Source: CAD feature listing. Evaluate the final solid. Frame: model axes, mm. A direction names the side the tool comes from. Coordinates: 2 decimals unless noted, no trailing zeros. Order: outer loops, then holes, each group sorted by start corner. A loop starts at its lowest first (then second) coordinate and runs counter-clockwise, first axis right, second up.
```python
from build123d import *

# Parameters (mm, degrees)
SKETCH1_W                 = 50.8
SKETCH1_H                 = 50.8
BOSS_EXTRUDE1_DEPTH       = 15.875
SKETCH2_R                 = 3.175
CUT_EXTRUDE1_DEPTH        = 59.973007597
TAP_DRILL_FOR_8_32_TAP1_D = 3.4544
SKETCH5_R                 = 3.81
CUT_EXTRUDE2_DEPTH        = 6.35


with BuildPart() as part:
    # Sketch1 → Boss-Extrude1 (new body)
    with BuildSketch(Plane(origin=(0, 0, 0), x_dir=(1, 0, 0), z_dir=(0, 1, 0))):
        Rectangle(SKETCH1_W, SKETCH1_H)
    extrude(amount=BOSS_EXTRUDE1_DEPTH)

    # Sketch2 → Cut-Extrude1 (cut, through all)
    with BuildSketch(Plane.XY.offset(25.4)):
        with Locations((-19.05, 7.9375)):
            Circle(SKETCH2_R)
        with Locations((0, 7.9375)):
            Circle(SKETCH2_R)
        with Locations((19.05, 7.9375)):
            Circle(SKETCH2_R)
    extrude(amount=-CUT_EXTRUDE1_DEPTH, mode=Mode.SUBTRACT)

    # Tap Drill for #8-32 Tap1 (through all)
    with Locations(Plane(origin=(0, 15.875, 0), x_dir=(1, 0, 0), z_dir=(0, 1, 0))):
        with Locations((-9.525, -12.7), (-9.525, 12.7), (9.525, 12.7), (9.525, -12.7)):
            Hole(TAP_DRILL_FOR_8_32_TAP1_D / 2)

    # Sketch5 → Cut-Extrude2 (cut)
    with BuildSketch(Plane(origin=(0, 15.875, 0), x_dir=(1, 0, 0), z_dir=(0, 1, 0))):
        with Locations(Location((-9.525, 12.7, 0), (0, 0, 270))):
            Circle(SKETCH5_R)
        with Locations(Location((9.525, 12.7, 0), (0, 0, 270))):
            Circle(SKETCH5_R)
        with Locations(Location((9.525, -12.7, 0), (0, 0, 270))):
            Circle(SKETCH5_R)
        with Locations(Location((-9.525, -12.7, 0), (0, 0, 270))):
            Circle(SKETCH5_R)
    extrude(amount=-CUT_EXTRUDE2_DEPTH, mode=Mode.SUBTRACT)


solid = part.part
```
1. Draft query along Z for faces 1 (the flat face through (0, 0, 0)), 2 (the flat face through (-0.4, 11.4, -25.4)), 3 (the flat face through (-11.2, 9.525, 11.8)). Return one class per face: +Z half, -Z half, draft (parallel to the pull), parting line (faces both ways), or undercut.
2. Section query A-A, the plane x = 0. Output: boundary loops of the cut face in (y, z) (1 decimal).
3. Section query D-D, the plane y = 13. Output: boundary loops of the cut face in (x, z) (3 decimals).
4. Section query B-B, the plane z = 12.7. Count the separate pieces of the cut face and the enclosed holes in it, plus the area to 3 significant figures.
5. Material intervals for line 1 along X through (y, z) = (12, 12.7) (3 decimals); line 2 along X through (y, z) = (10.5, 8); line 3 along Y through (x, z) = (19, -10) (3 decimals), sorted ascending.
6. Section query C-C, the plane y = 7.25. Output: boundary loops of the cut face in (x, z) (3 decimals).
7. Access query for faces 4 (the cylindrical face through (9.693, 12.744, -16.506)), 5 (the cylindrical face through (-9.151, 4.696, -11.014)). Directions: +Z, -Z, +X, -X, +Y, -Y. A direction counts if a zero-diameter tool reaches every point of the face in a straight line with its end or side. Return the directions, or none.
8. Contact query for flat-ended pins moving along their axis: P1, Ø1.5, axis at x = 13, z = 17, coming from the -Y side; P2, Ø6, axis at x = -9.525, z = -12.7, coming from the +Y side (3 decimals). Output: stop coordinate, or through.
Answer key:
1. face 1: draft
1. face 2: -Z half
1. face 3: undercut
2. outline: (0, -25.4) - (4.8, -25.4) - (4.8, 25.4) - (0, 25.4) - close; (11.1, -25.4) - (15.9, -25.4) - (15.9, 25.4) - (11.1, 25.4) - close
3. outline: (-25.4, -25.4) - (25.4, -25.4) - (25.4, 25.4) - (-25.4, 25.4) - close; hole circle Ø7.62 at (-9.525, -12.7); hole circle Ø7.62 at (-9.525, 12.7); hole circle Ø7.62 at (9.525, -12.7); hole circle Ø7.62 at (9.525, 12.7)
4. separate pieces: 3
4. enclosed holes: 3
4. area: 549 mm2
5. line 1: x = -25.4 to -13.335, -5.715 to 5.715, 13.335 to 25.4
5. line 2: x = -25.4 to -20.92, -17.18 to -1.87, 1.87 to 17.18, 20.92 to 25.4
5. line 3: y = 0 to 4.763, 11.112 to 15.875
6. outline: (-25.4, -25.4) - (-22.15, -25.4) - (-22.15, 25.4) - (-25.4, 25.4) - close; (-15.95, -25.4) - (-3.1, -25.4) - (-3.1, 25.4) - (-15.95, 25.4) - close; (3.1, -25.4) - (15.95, -25.4) - (15.95, 25.4) - (3.1, 25.4) - close; (22.15, -25.4) - (25.4, -25.4) - (25.4, 25.4) - (22.15, 25.4) - close; hole circle Ø3.454 at (-9.525, -12.7); hole circle Ø3.454 at (-9.525, 12.7); hole circle Ø3.454 at (9.525, -12.7); hole circle Ø3.454 at (9.525, 12.7)
7. face 4: +Y
7. face 5: +Y, -Y
8. P1: stops at y = 0
8. P2: stops at y = 9.525
